Design review of the part built by this model. Coordinates are the model's own, in mm. Coordinates: 2 decimals unless noted, no trailing zeros. Write each loop counter-clockwise with the first axis right and the second up, starting at its lowest first coordinate (ties: lowest second). Pieces come first, ordered by that corner, then holes. Notation, with made-up numbers: M 40,38 L 49,38 A19 cw 49,74 Z; hole C 23.5,52.25 d11. An arc over 180 degrees is marked long. Return JSON: item names as keys, results as strings. Group by question number.
Autodesk Inventor part; units mm, degrees
ref_plane "YZ Plane" through (0, 0, 0) normal (1, 0, 0) x (0, 1, 0)
ref_plane "XZ Plane" through (0, 0, 0) normal (0, 1, 0) x (-1, 0, 0)
ref_plane "XY Plane" through (0, 0, 0) normal (0, 0, 1) x (1, 0, 0)
sketch "Sketch1" plane through (0, 0, 0) normal (0, 1, 0) x (-1, 0, 0)
  line L0 (0, 0) -> (-139.7, 0)
  line L1 (-139.7, 0) -> (-139.7, -238.125)
  line L2 (-139.7, -238.125) -> (0, -238.125)
  line L3 (0, -238.125) -> (0, 0)
  line L4 (-3.175, -3.175) -> (-136.525, -3.175)
  line L5 (-136.525, -3.175) -> (-136.525, -234.95)
  line L6 (-136.525, -234.95) -> (-3.175, -234.95)
  line L7 (-3.175, -234.95) -> (-3.175, -3.175)
  line L8 (0, -238.125) -> (-139.7, -238.125)
  line L9 (-69.85, -238.125) -> (-59.69, -238.125)
  line L10 (-59.69, -238.125) -> (-80.01, -238.125)
  line L11 (-80.01, -234.95) -> (-59.69, -234.95)
  line L12 (-69.85, -238.125) -> (-69.85, -234.95)
  line L13 (-69.85, -238.125) -> (-44.45, -238.125)
  line L14 (-44.45, -238.125) -> (-95.25, -238.125)
  line L15 (-95.25, -238.125) -> (-95.25, -234.95)
  line L16 (-95.25, -234.95) -> (-44.45, -234.95)
  line L17 (-44.45, -234.95) -> (-44.45, -238.125)
  line L18 (-44.45, -238.125) -> (-95.25, -238.125)
  dimension "d0" = 139.7
  dimension "d1" = 238.125
  dimension "d2" = 3.175
  dimension "d45" = 25.4
  dimension "d46" = 50.8
extrude "Extrusion1" add sketch "Sketch1" along normal blind 3.175 contours L3 L2 L17 L6 L7 L4 L5 L15 L1 L0
sketch "Sketch2" plane through (0, 3.175, 0) normal (0, 1, 0) x (1, 0, 0)
  line L0 (0, 238.125) -> (0, 0)
  line L1 (139.7, 238.125) -> (0, 238.125)
  line L2 (0, 0) -> (139.7, 0)
  line L3 (139.7, 0) -> (139.7, 238.125)
  line L4 (139.7, 238.125) -> (0, 238.125)
  line L5 (0, 238.125) -> (0, 0)
  line L6 (139.7, -3.175) -> (0, -3.175)
  line L7 (-3.175, 0) -> (-3.175, 238.125)
  line L8 (0, 241.3) -> (139.7, 241.3)
  line L9 (142.875, 238.125) -> (142.875, 0)
  arc A0 (0, 241.3) -> (-3.175, 238.125) centre (0, 238.125) ccw
  arc A1 (-3.175, 0) -> (0, -3.175) centre (0, 0) ccw
  arc A2 (139.7, -3.175) -> (142.875, 0) centre (139.7, 0) ccw
  arc A3 (142.875, 238.125) -> (139.7, 241.3) centre (139.7, 238.125) ccw
  line L10 (136.525, 3.175) -> (3.175, 3.175)
  line L11 (139.7, 234.95) -> (3.175, 234.95)
  line L12 (3.175, 234.95) -> (3.175, 3.175)
  line L13 (3.175, 3.175) -> (139.7, 3.175)
  line L14 (139.7, 3.175) -> (139.7, 234.95)
  point P0 (80.01, 238.125)
  point P1 (139.7, 3.175)
  point P2 (139.7, 234.95)
  dimension "d7" = 3.175
extrude "Extrusion2" add sketch "Sketch2" along normal blind 3.175 contours L1 L3 L11 L12 L10 L13 L2 L0 | L3 L13 L10 L12 L11 | L6 A1 L7 A0 L8 A3 L9 A2
sketch "Sketch3" plane through (142.875, 3.175, 0) normal (1, 0, 0) x (0, 0, -1)
  line L0 (-3.175, 3.175) -> (241.3, 3.175)
  line L1 (0, 3.175) -> (238.125, 3.175)
  line L2 (119.0625, 3.175) -> (119.0625, 38.1)
  line L3 (119.0625, 38.1) -> (42.8625, 38.1)
  line L4 (119.0625, 38.1) -> (169.8625, 38.1)
  line L5 (-3.175, 3.175) -> (42.8625, 38.1)
  line L6 (169.8625, 38.1) -> (241.3, 3.175)
  line L7 (43.9305, 34.925) -> (119.0625, 34.925)
  line L8 (119.0625, 34.925) -> (169.1279, 34.925)
  line L9 (169.1279, 34.925) -> (227.5768, 6.35)
  line L10 (227.5768, 6.35) -> (6.2635, 6.35)
  line L11 (6.2635, 6.35) -> (43.9305, 34.925)
  point P0 (0, -3.175)
  dimension "d10" = 34.925
  dimension "d11" = 76.2
  dimension "d12" = 50.8
  dimension "d13" = 3.175
extrude "Extrusion3" add sketch "Sketch3" against normal blind 146.05 contours L5 L3 L2 L7 L11 L10 L0 | L2 L10 L9 L8 L4 L6 L0
sketch "Sketch4" plane through (0, 0, 0) normal (0, -1, 0) x (1, 0, 0)
  line L0 (0, 0) -> (139.7, 0)
  line L1 (0, -238.125) -> (139.7, -238.125)
  line L2 (0, 0) -> (139.7, 0)
  line L3 (139.7, 0) -> (139.7, -238.125)
  line L4 (139.7, -238.125) -> (0, -238.125)
  line L5 (0, -238.125) -> (0, 0)
  line L6 (136.525, -234.95) -> (136.525, -3.175)
  line L7 (136.525, -3.175) -> (3.175, -3.175)
  line L8 (3.175, -3.175) -> (3.175, -234.95)
  line L9 (3.175, -234.95) -> (136.525, -234.95)
extrude "Extrusion4" cut sketch "Sketch4" against normal blind 36.83 contours L9 L8 L7 L6
sketch "Sketch7" plane through (142.875, 41.275, -42.8625) normal (0, 1, 0) x (1, 0, 0)
  line L0 (-146.05, -36.599) -> (-146.05, 184.7143)
  line L1 (-146.05, 0) -> (0, 0)
  line L2 (0, 0) -> (0, 127)
  line L3 (0, 127) -> (-146.05, 127)
  line L4 (-146.05, 127) -> (-146.05, 0)
  line L5 (-139.7, 120.65) -> (-6.35, 120.65)
  line L6 (-6.35, 120.65) -> (-6.35, 6.35)
  line L7 (-6.35, 6.35) -> (-139.7, 6.35)
  line L8 (-139.7, 6.35) -> (-139.7, 120.65)
  point P0 (-142.875, -42.8625)
  dimension "d36" = 6.35
extrude "Extrusion6" cut sketch "Sketch7" against normal blind 36.83 contours L5 L6 L7 L8
fillet "Fillet1" radius 3.175 1 edges at (142.875, 23.8125, -19.8437)
fillet "Fillet2" radius 3.175 1 edges at (142.875, 23.8125, -205.5813)
fillet "Fillet3" radius 3.175 2 edges at (-3.175, 23.8125, -19.8437) (-3.175, 23.8125, -205.5813)
sketch "Sketch8" plane through (0, 0, 0) normal (0, -1, 0) x (1, 0, 0)
  line L0 (0, 0) -> (139.7, 0)
  line L1 (139.7, 0) -> (139.7, -238.125)
  line L2 (139.7, -238.125) -> (0, -238.125)
  line L3 (0, -238.125) -> (0, 0)
  line L4 (0.635, -237.49) -> (139.065, -237.49)
  line L5 (139.065, -237.49) -> (139.065, -0.635)
  line L6 (139.065, -0.635) -> (0.635, -0.635)
  line L7 (0.635, -0.635) -> (0.635, -237.49)
  dimension "d42" = 0.635
extrude "Extrusion7" cut sketch "Sketch8" against normal blind 3.175
properties part number "TopLid_3DPrint"
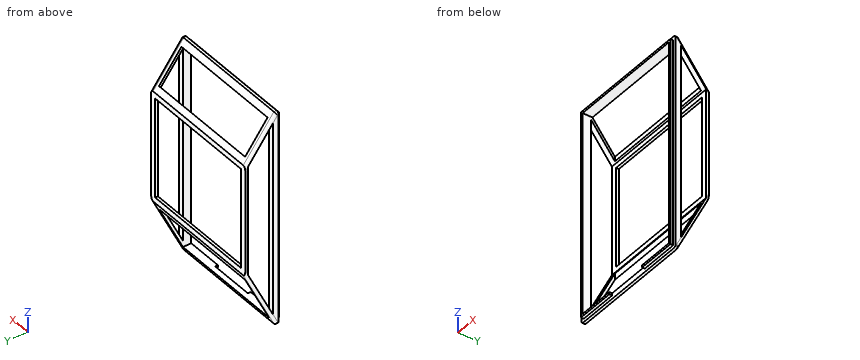
Item 1: For line 1 (X direction, y = 2, z = -184) (3 decimals); line 2 (X direction, y = 6, z = -71.5) (3 decimals); line 3 (Z direction, x = 123.5, y = 4.5) (3 decimals), list the stretches that pass through material, from the lowest coordinate up.
Item 2: Add section A-A (x = 66). Count the separate pieces of the cut face and the enclosed holes in it, plus the area to 3 significant figures.
Item 3: For pin 1 (4 mm diameter, centred on x = 43.5, z = -40, fed in from -Y); pin 2 (2.5 mm diameter, centred on x = 58.5, y = 1, fed in from +Z) (3 decimals); pin 3 (5 mm diameter, centred on x = 76.5, y = 10, fed in from -Z), all flat-tipped, find the tip position at first contact; note any pin that passes through.
Item 4: Add section B-B (z = -53). Write out the cut boundary in (x, y) (3 decimals).
Geometry check:
{
 "1": {"line 1": "0.635 to 3.175, 136.525 to 139.065", "line 2": "-3.175 to 3.175, 136.525 to 142.875", "line 3": "-241.3 to -234.95, -3.175 to 3.175"},
 "2": {"separate pieces": "4", "enclosed holes": "0", "area": "147 mm^2"},
 "3": {"pin 1": "y = 36.83", "pin 2": "z = -0.635", "pin 3": "z = -238.95"},
 "4": {"outline": "M -3.175,3.175 L 0.635,3.175 L 0.635,0 L 3.175,0 L 3.175,9.525 L -3.175,9.525 Z; M -3.175,38.1 L 3.175,38.1 L 3.175,41.275 L -3.175,41.275 Z; M 136.525,0 L 139.065,0 L 139.065,3.175 L 142.875,3.175 L 142.875,9.525 L 136.525,9.525 Z; M 136.525,38.1 L 142.875,38.1 L 142.875,41.275 L 136.525,41.275 Z"}
}
